from build123d import *

# Parameters (mm, degrees)
SALIENTE_EXTRUIR1_DEPTH = 10
SALIENTE_EXTRUIR2_DEPTH = 6.2
CORTAR_EXTRUIR1_REACH   = 12
CROQUIS3_R              = 1.6
CORTAR_EXTRUIR2_DEPTH   = 3


with BuildPart() as part:
    # Croquis1 → Saliente-Extruir1 (new body)
    with BuildSketch(Plane.XY):
        Polygon((0, 0), (19, 0), (19, 3), (9, 3), (9, 29.7), (19, 29.7), (19, 35.9), (0, 35.9), align=None)
    extrude(amount=SALIENTE_EXTRUIR1_DEPTH)

    # Croquis2 → Saliente-Extruir2 (add)
    with BuildSketch(Plane.XY.offset(10)):
        Polygon((9, 29.7), (0, 29.7), (0, 0), (19, 0), (19, 3), (9, 3), align=None)
    extrude(amount=SALIENTE_EXTRUIR2_DEPTH)

    # Croquis3 → Cortar-Extruir1 (cut, up to next)
    with BuildSketch(Plane.XY.offset(10), mode=Mode.PRIVATE) as cortar_extruir1_sk1:
        with Locations((4.3, 32.8)):
            Circle(CROQUIS3_R)
    cortar_extruir1_tool1 = extrude(cortar_extruir1_sk1.sketch, amount=-CORTAR_EXTRUIR1_REACH, mode=Mode.PRIVATE) & part.part
    add(cortar_extruir1_tool1.solids().sort_by_distance((4.3, 32.8, 10))[0], mode=Mode.SUBTRACT)

    # Croquis4 → Cortar-Extruir2 (cut)
    with BuildSketch(Plane(origin=(0, 0, 0), x_dir=(-1, 0, 0), z_dir=(0, 0, -1))):
        Polygon((-2.654551733, 35.65), (-5.945448267, 35.65), (-7.590896534, 32.8), (-5.945448267, 29.95), (-2.654551733, 29.95), (-1.009103466, 32.8), align=None)
    extrude(amount=-CORTAR_EXTRUIR2_DEPTH, mode=Mode.SUBTRACT)


solid = part.part
Source: CAD feature listing. Evaluate the final solid. Frame: model axes, mm. A direction names the side the tool comes from. Give positions to 0.01 mm unless a question says otherwise; leave off trailing zeros. Loops run counter-clockwise (first coordinate to the right, second up) from the corner with the lowest first, then second, coordinate; pieces in that order, holes last. Notation, with made-up numbers: (79.5, 14) -> (115.5, 14) arc R21 cw to (115.5, 20) -> close; hole circle Ø7 at (63, 13.25). An arc over 180 degrees is marked (long way). Use a Markdown table: item, result. Add a question column.
1) Line query: line 1 along Y through (x, z) = (4.3, 6); line 2 along X through (y, z) = (22, 5.25); line 3 along Y through (x, z) = (16.75, 5). Output: solid intervals per line, ascending. Write a range as [from, to].
2) Section query C-C, the plane y = 32. Return the cut outline in (x, z).
3) Section query A-A, the plane x = 11. Return the cut outline in (y, z), then the cut area to 3 significant figures.
4) Section query D-D, the plane x = 8. Return the cut outline in (y, z), then the cut area to 3 significant figures.
5) First-contact query: pin 1 (7 mm diameter, centred on x = 8.5, y = 33.5, fed in from +Z); pin 2 (5 mm diameter, centred on y = 21, z = 12, fed in from +X); pin 3 (3 mm diameter, centred on x = 4, y = 33, fed in from -Z); pin 4 (2 mm diameter, centred on x = 16.5, y = 27.5, fed in from +Z). Flat tips, straight axial feed; report the tip coordinate or a pass-through.
6) Section query B-B, the plane z = 1.75. Return the cut outline in (x, y), then the cut area to 3 significant figures.
7) Pull-direction query (Y, two-part tool) for faces 5 (the face through (9, 16, 8)), 6 (the face through (7, 18, 0)), 7 (the face through (5, 29.7, 13)), 8 (the face through (6.76, 34.24, 1.48)); classes: +Y half, -Y half, draft (parallel to the pull), parting line (faces both ways), or undercut.
8) Reachability of faces 1 (the face through (14, 3, 8)), 2 (the face through (9, 33, 10)), 3 (the face through (4, 29.95, 1)), 4 (the face through (9, 0, 8)) from +Z, -Z, +X, -X, +Y, -Y: full face, straight path, thin tool, end or side. Return the list, or none.
Numbers:
| question | item | result |
|---|---|---|
| 1 | line 1 | y = [0, 31.2], [34.4, 35.9] |
| 1 | line 2 | x = [0, 9] |
| 1 | line 3 | y = [0, 3], [29.7, 35.9] |
| 2 | outline | (0, 0) -> (1.47, 0) -> (1.47, 3) -> (2.91, 3) -> (2.91, 10) -> (0, 10) -> close; (5.69, 3) -> (7.13, 3) -> (7.13, 0) -> (19, 0) -> (19, 10) -> (5.69, 10) -> close |
| 3 | outline | (0, 0) -> (3, 0) -> (3, 16.2) -> (0, 16.2) -> close; (29.7, 0) -> (35.9, 0) -> (35.9, 10) -> (29.7, 10) -> close |
| 3 | area | 111 mm2 |
| 4 | outline | (0, 0) -> (35.9, 0) -> (35.9, 10) -> (29.7, 10) -> (29.7, 16.2) -> (0, 16.2) -> close |
| 4 | area | 543 mm2 |
| 5 | pin 1 | stops at z = 10 |
| 5 | pin 2 | stops at x = 9 |
| 5 | pin 3 | stops at z = 3 |
| 5 | pin 4 | passes through |
| 6 | outline | (0, 0) -> (19, 0) -> (19, 3) -> (9, 3) -> (9, 29.7) -> (19, 29.7) -> (19, 35.9) -> (0, 35.9) -> close; hole (1.01, 32.8) -> (2.65, 29.95) -> (5.95, 29.95) -> (7.59, 32.8) -> (5.95, 35.65) -> (2.65, 35.65) -> close |
| 6 | area | 387 mm2 |
| 7 | face 5 | undercut |
| 7 | face 6 | draft |
| 7 | face 7 | +Y half |
| 7 | face 8 | undercut |
| 8 | face 1 | +Z, -Z, +X |
| 8 | face 2 | +Z, +X, -X, +Y |
| 8 | face 3 | -Z |
| 8 | face 4 | +Z, -Z, +X, -X, -Y |
